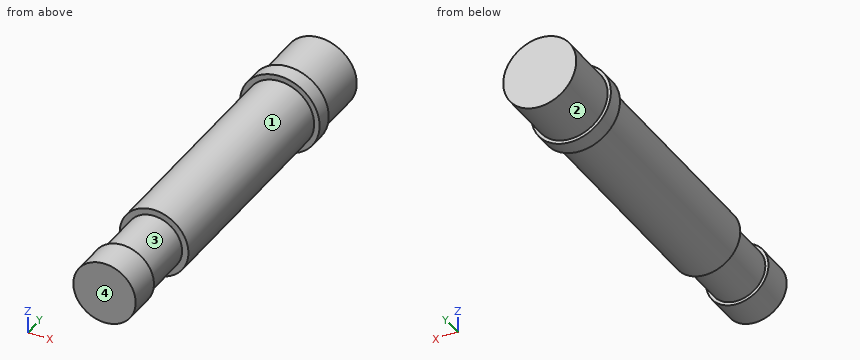
Autodesk Inventor part; units mm, degrees
ref_plane "YZ Plane" through (0, 0, 0) normal (1, 0, 0) x (0, 1, 0)
ref_plane "XZ Plane" through (0, 0, 0) normal (0, 1, 0) x (-1, 0, 0)
ref_plane "XY Plane" through (0, 0, 0) normal (0, 0, 1) x (1, 0, 0)
sketch "Sketch1" plane through (0, 0, 0) normal (0, 0, 1) x (1, 0, 0)
  line L0 (0, 0) -> (-13.97, 0)
  line L1 (-13.97, 0) -> (-13.97, -21.844)
  line L2 (-13.97, -21.844) -> (-15.24, -21.844)
  line L3 (-15.24, -21.844) -> (-15.24, -28.194)
  line L4 (-15.24, -28.194) -> (-13.1445, -28.194)
  line L5 (-13.1445, -28.194) -> (-13.1445, -115.824)
  line L6 (-13.1445, -115.824) -> (-10.7315, -115.824)
  line L7 (-10.7315, -115.824) -> (-10.7315, -137.668)
  line L8 (-10.7315, -137.668) -> (-11.938, -137.668)
  line L9 (-11.938, -137.668) -> (-11.938, -150.368)
  line L10 (-11.938, -150.368) -> (0, -150.368)
  line L11 (0, -150.368) -> (0, 0)
  dimension "d0" = 21.844
  dimension "d1" = 13.97
  dimension "d2" = 6.35
  dimension "d3" = 15.24
  dimension "d4" = 13.1445
  dimension "d5" = 87.63
  dimension "d7" = 10.7315
  dimension "d8" = 21.844
  dimension "d9" = 11.938
  dimension "d10" = 12.7
revolve "Revolution1" add sketch "Sketch1" angle 360 about axis through (0, -150.368, 0) along (0, 1, 0)
equation "\"d0\" = endLength"
equation "\"d1\" = endRadius"
equation "\"d2\" = bandLength"
equation "\"d3\" = bandRadius"
equation "\"d4\" = mainBodyRadius"
equation "\"d5\" = mainBodyLength"
equation "\"d7\" = eyepieceEndRadius"
equation "\"d8\" = endLength"
equation "\"d9\" = eyepieceRadius"
equation "\"d10\" = eyepieceLength"
equation "\"endRadius\" = 13.97"
equation "\"bandRadius\" = 15.24"
equation "\"mainBodyRadius\" = 13.1445"
equation "\"eyepieceEndRadius\" = 10.7315"
equation "\"eyepieceRadius\" = 11.938"
equation "\"endLength\" = 21.844"
equation "\"bandLength\" = 6.35"
equation "\"mainBodyLength\" = 87.63"
equation "\"eyepieceEndLength\" = 13.97"
equation "\"eyepieceLength\" = 12.7"
properties part number "celestronFinder"
Here's how the part is built. I have some questions about the finished solid (model axes, mm). Face numbers are marked on the shaded views. A direction names the side the tool comes from. Give positions to 0.01 mm unless a question says otherwise; leave off trailing zeros. Order: outer loops, then holes, each group sorted by start corner. A loop starts at its lowest first (then second) coordinate and runs counter-clockwise, first axis right, second up. Notation, with made-up numbers: M -38.75,43.5 L 4.25,43.5 A19 cw 4.25,69.5 Z; hole C 25,57.25 d9. An arc over 180 degrees is marked long. Use a Markdown table: item, result. Add a question column.
1. Suppose I cut it at C-C (y = -126). List the corners of the cut face in (x, z) for me, and give its area (3 significant figures).
2. For pin 1 Ø2 at (y, z) = (-97.5, -8) entering from +X; pin 2 Ø1.5 at (x, y) = (-9, -118.5) entering from -Z; pin 3 Ø8 at (x, y) = (-4.5, -30.5) entering from +Z, each with a flat end and sliding along its axis, tell me the tip position at first contact or that it passes through.
3. I need wall thicknesses on probe 1 along Y at (x, z) = (9, 9.5); probe 2 along Z at (x, y) = (5.5, -106); probe 3 along Y at (x, z) = (-11, -3). Which ranges of each line are inside material? Lowest first, please. Write a range as from..to.
4. Suppose I cut it at A-A (x = 0). List the corners of the cut face in (y, z) for me, and give its area (3 significant figures).
5. Suppose I cut it at B-B (z = 0). List the corners of the cut face in (x, y) for me.
6. On a 3-axis mill with a long thin cutter (end or side, diameter ignored), from which of +Z, -Z, +X, -X, +Y, -Y can I reach the whole of each face in a straight line? I mean the marked faces 1, 2, 3 and 4. Say none if no direction works.
Results list:
| question | item | result |
|---|---|---|
| 1 | outline | C 0,0 d21.46 |
| 1 | area | 362 mm² |
| 2 | pin 1 | stops at x = 11.13 |
| 2 | pin 2 | stops at z = -6.86 |
| 2 | pin 3 | stops at z = 15.19 |
| 3 | probe 1 | y = -115.82..0 |
| 3 | probe 2 | z = -11.94..11.94 |
| 3 | probe 3 | y = -150.37..-137.67, -115.82..0 |
| 4 | outline | M -150.37,-11.94 L -137.67,-11.94 L -137.67,-10.73 L -115.82,-10.73 L -115.82,-13.14 L -28.19,-13.14 L -28.19,-15.24 L -21.84,-15.24 L -21.84,-13.97 L 0,-13.97 L 0,13.97 L -21.84,13.97 L -21.84,15.24 L -28.19,15.24 L -28.19,13.14 L -115.82,13.14 L -115.82,10.73 L -137.67,10.73 L -137.67,11.94 L -150.37,11.94 Z |
| 4 | area | 3,880 mm² |
| 5 | outline | M -15.24,-28.19 L -13.14,-28.19 L -13.14,-115.82 L -10.73,-115.82 L -10.73,-137.67 L -11.94,-137.67 L -11.94,-150.37 L 11.94,-150.37 L 11.94,-137.67 L 10.73,-137.67 L 10.73,-115.82 L 13.14,-115.82 L 13.14,-28.19 L 15.24,-28.19 L 15.24,-21.84 L 13.97,-21.84 L 13.97,0 L -13.97,0 L -13.97,-21.84 L -15.24,-21.84 Z |
| 6 | face 1 | -Y |
| 6 | face 2 | +Y |
| 6 | face 3 | none |
| 6 | face 4 | +Z, -Z, +X, -X, -Y |
